The listing builds one solid part. Answer for the finished solid, in the listing's coordinates (mm). A direction names the side the tool comes from. Round coordinates to 2 decimals unless told otherwise and drop trailing zeros. Write each loop counter-clockwise with the first axis right and the second up, starting at its lowest first coordinate (ties: lowest second). Pieces come first, ordered by that corner, then holes. Notation, with made-up numbers: M -36.5,71.5 L -19.5,71.5 A23 cw -19.5,95.5 Z; hole C 4,43.25 d8. An arc over 180 degrees is marked long. Write each question's results on one line, items separated by ' | '.
from build123d import *

# Parameters (mm, degrees)
CUT_EXTRUDE1_DEPTH = 1.04


with BuildPart() as part:
    # Sketch1 → Revolve1 (revolve)
    with BuildSketch(Plane(origin=(0, 0, 0), x_dir=(1, 0, 0), z_dir=(0, 1, 0))):
        with BuildLine():
            Line((0, 0), (17.65, 0))
            Line((17.65, 0), (17.65, 1.5))
            Line((17.65, 1.5), (1.65, 1.5))
            Line((1.65, 1.5), (1.65, 2.85))
            Line((1.65, 2.85), (1.5, 2.85))
            ThreePointArc((1.5, 2.85), (0.439339828, 2.410660172), (0, 1.35))
            Line((0, 1.35), (0, 0))
        make_face()
    revolve(axis=Axis((0, 0, 0), (-1, 0, 0)))

    # Sketch2 → Cut-Extrude1 (cut)
    with BuildSketch(Plane.ZY):
        Polygon((1.154700538, 0), (0.577350269, 1), (-0.577350269, 1), (-1.154700538, 0), (-0.577350269, -1), (0.577350269, -1), align=None)
    extrude(amount=-CUT_EXTRUDE1_DEPTH, mode=Mode.SUBTRACT)


solid = part.part
1) Find the intervals of material crossed by line 1 (Z direction, x = 15.5, y = -0.65); line 2 (X direction, y = 0.95, z = 0.1); line 3 (Y direction, x = 7, z = -0.1), in increasing order.
Return value:
line 1: -1.35 to 1.35 | line 2: 1.04 to 17.65 | line 3: -1.5 to 1.5
2) The mould has two halves that part along Z. Classify faces 1 (the face through (17.65, 0, 0)), 2 (the face through (9.54, -0.07, 1.5)), 3 (the face through (0.51, -0.49, -0.87)): +Z half, -Z half, draft (parallel to the pull), parting line (faces both ways), or undercut.
Return value:
face 1: draft | face 2: parting line | face 3: undercut
3) A tool of negligible diameter and unlimited length cuts with its end or side. For faces 4 (the face through (1.65, 1.2, 1.2)), 5 (the face through (0.51, 0.49, 0.87)), from which of +Z, -Z, +X, -X, +Y, -Y can it reach the whole face along a straight path? Write none if from no direction.
Return value:
face 4: +X | face 5: -X
4) Section A-A (x = 13.5) is taken. Determine the outline of the cut face in (y, z), then the cut area to 3 significant figures.
Return value:
outline: C 0,0 d3 | area: 7.07 mm²
5) Each of these flat-tipped pins is pushed along its axis until it touches: pin 1 (0.8 mm diameter, centred on x = 0.5, z = -0.5, fed in from -Y); pin 2 (1 mm diameter, centred on y = 2, z = 0, fed in from -X); pin 3 (3 mm diameter, centred on x = 5.5, z = -2, fed in from -Y). Where does it stop, or does it pass through?
Return value:
pin 1: y = -2.69 | pin 2: x = 0.01 | pin 3: y = -1.41
